from build123d import *

# Parameters (mm, degrees)
F0_W        = 99.15
F0_H        = 9.75
F1_DEPTH    = 4.75
F2_R        = 2.5
F3_DEPTH    = 4.751
F4_W        = 12
F4_H        = 7
F5_DEPTH    = 25.4
F6_T1_DEPTH = 37.9
F7_R        = 1.5
F8_R        = 1.75
F9_W        = 59
F9_H        = 4
F10_DEPTH   = 25
F11_R       = 1.5


# Not quite as in the source:
# - a fillet or chamfer that OpenCascade refuses, or shapes differently, is made with other operations: its cross-section is extruded or revolved along the edge and cut away or added


with BuildPart() as f1:
    # F0 (on Top) → F1 (new body)
    with BuildSketch(Plane.XY):
        Rectangle(F0_W, F0_H)
    extrude(amount=F1_DEPTH)

    # F2 (on face) → F3 (cut, through all)
    with BuildSketch(Plane.XY.offset(4.75)):
        with Locations((42.075, 0)):
            Circle(F2_R)
    extrude(amount=-F3_DEPTH, mode=Mode.SUBTRACT)

    # F4 (on face) → F5 (join)
    with BuildSketch(Plane.XY.offset(4.75)):
        with Locations((23.525, 0)):
            Rectangle(F4_W, F4_H)
    extrude(amount=F5_DEPTH)

    # F6: fillet of radius 5 on 4 edges, made by hand

    # F6_s2 → F6_t1 (cut)
    with BuildSketch(Plane.XY.offset(4.75)):
        with BuildLine():
            ThreePointArc((22.525, 3.5), (18.9894660941, 2.0355339059), (17.525, -1.5))
            Line((17.525, -1.5), (17.525, 3.5))
            Line((17.525, 3.5), (22.525, 3.5))
        make_face()
        with BuildLine():
            ThreePointArc((17.525, 1.5), (18.9894660941, -2.0355339059), (22.525, -3.5))
            Line((22.525, -3.5), (17.525, -3.5))
            Line((17.525, -3.5), (17.525, 1.5))
        make_face()
        with BuildLine():
            ThreePointArc((29.525, -1.5), (28.0605339059, 2.0355339059), (24.525, 3.5))
            Line((24.525, 3.5), (29.525, 3.5))
            Line((29.525, 3.5), (29.525, -1.5))
        make_face()
        with BuildLine():
            ThreePointArc((29.525, 1.5), (28.0605339059, -2.0355339059), (24.525, -3.5))
            Line((24.525, -3.5), (29.525, -3.5))
            Line((29.525, -3.5), (29.525, 1.5))
        make_face()
    extrude(amount=F6_T1_DEPTH, mode=Mode.SUBTRACT)

    # F7
    f7_edges = [f1.edges().sort_by_distance(p)[0] for p in [
        (-49.575, 4.875, 2.375),
        (-49.575, -4.875, 2.375),
        (-49.575, 0, 0),
        (-49.575, 0, 4.75),
        (49.575, -4.875, 2.375),
        (49.575, 4.875, 2.375),
        (49.575, 0, 0),
        (49.575, 0, 4.75),
    ]]
    fillet(f7_edges, radius=F7_R)

    # F8
    f8_edges = [f1.edges().sort_by_distance(p)[0] for p in [
        (23.525, -3.5, 30.15),
        (19.56696, -2.531129, 30.15),
        (19.56696, 2.531129, 30.15),
        (23.525, 3.5, 30.15),
        (27.48304, 2.531129, 30.15),
        (27.48304, -2.531129, 30.15),
    ]]
    fillet(f8_edges, radius=F8_R)

    # F9 (on face) → F10 (cut)
    with BuildSketch(Plane.XY.offset(4.75)):
        with Locations((-16, 0)):
            Rectangle(F9_W, F9_H)
    extrude(amount=-F10_DEPTH, mode=Mode.SUBTRACT)

    # F11
    f11_edges = [f1.edges().sort_by_distance(p)[0] for p in [
        (-16, 2, 4.75),
        (-45.5, 0, 4.75),
        (-16, -2, 4.75),
        (13.5, 0, 4.75),
        (13.5, 0, 0),
        (-16, 2, 0),
        (-16, -2, 0),
        (-45.5, 0, 0),
    ]]
    fillet(f11_edges, radius=F11_R)


solid = f1.part
Could you check a few things on this model? Use its own coordinates, in mm. A direction names the side the tool comes from. Give positions to 0.01 mm unless a question says otherwise; leave off trailing zeros. Order: outer loops, then holes, each group sorted by start corner. A loop starts at its lowest first (then second) coordinate and runs counter-clockwise, first axis right, second up. Notation, with made-up numbers: M -15,4.5 L 38,4.5 A5 cw 38,11.5 Z; hole C 72,44.5 d9. An arc over 180 degrees is marked long. One line per question, with ' | ' between items.
1. We'd pull the mould along X, two halves only. Please class faces 5 (the face through (24, -3.5, 16)), 6 (the face through (-49.575, 0, 2)), 7 (the face through (13.5, 0, 2)): +X half, -X half, draft (parallel to the pull), parting line (faces both ways), or undercut.
Results:
face 5: draft | face 6: -X half | face 7: undercut
2. I want a section at B-B (z = 21). List the corners of the cut face in (x, y) for me (3 decimals), and give its area (3 significant figures).
Results:
outline: M 17.755,0 A5 ccw 22.525,-3.5 L 24.525,-3.5 A5 ccw 29.295,0 A5 ccw 24.525,3.5 L 22.525,3.5 A5 ccw Z | area: 63.0 mm²
3. For faces 1 (the face through (27.519, -2.505, 16.409)), 2 (the face through (27.519, 2.505, 16.409)), 3 (the face through (24, 3.5, 16)), 4 (the face through (-45.5, 0, 2)), which set-ups out of +Z, -Z, +X, -X, +Y, -Y let a thin tool reach every point of the face, with its end or its side?
Results:
face 1: +Z, +X, -Y | face 2: +Z, +X, +Y | face 3: +Z, +X, -X, +Y | face 4: +Z, -Z
4. I want a section at C-C (x = 41.5). List the corners of the cut face in (y, z) for me (3 decimals), and give its area (3 significant figures).
Results:
outline: M -4.875,0 L -2.433,0 L -2.433,4.75 L -4.875,4.75 Z; M 2.433,0 L 4.875,0 L 4.875,4.75 L 2.433,4.75 Z | area: 23.2 mm²
5. If I drill on line 1 (X direction, y = -1.5, z = 4) (3 decimals); line 2 (Z direction, x = 30.5, y = 3.75); line 3 (Z direction, x = -6.5, y = -3.25), over which ranges is the centre line in solid material (lowest first)?
Results:
line 1: -49.374 to -45.701, 13.701 to 40.075, 44.075 to 49.374 | line 2: 0 to 4.75 | line 3: 0.02 to 4.73
6. I'm going to push flat-ended pins straight in: pin 1 (2 mm diameter, centred on x = 23, z = 21.5, fed in from +Y); pin 2 (3 mm diameter, centred on x = 14.5, y = 0, fed in from +Z); pin 3 (1.5 mm diameter, centred on y = 3, z = 24, fed in from -X); pin 4 (4 mm diameter, centred on x = 42.075, y = 0, fed in from -Z). Where does each tip first touch, or does it pass through?
Results:
pin 1: y = 3.5 | pin 2: z = 4.75 | pin 3: x = 19.22 | pin 4: through
7. I want a section at A-A (x = -22.5). List the corners of the cut face in (y, z) for me (3 decimals).
Results:
outline: M -4.875,0 L -3.5,0 A1.5 ccw -2,1.5 L -2,3.25 A1.5 ccw -3.5,4.75 L -4.875,4.75 Z; M 2,1.5 A1.5 ccw 3.5,0 L 4.875,0 L 4.875,4.75 L 3.5,4.75 A1.5 ccw 2,3.25 Z
